Source: CAD feature listing. Evaluate the final solid. Frame: model axes, mm. A direction names the side the tool comes from. Coordinates: 2 decimals unless noted, no trailing zeros. Order: outer loops, then holes, each group sorted by start corner. A loop starts at its lowest first (then second) coordinate and runs counter-clockwise, first axis right, second up.
```python
from build123d import *

# Parameters (mm, degrees)
TOP_CHAMFER_SIZE   = 1.5
BACK_CHAMFER_SIZE  = 2
BACK_CHAMFER_SIZE2 = 11.342563639
WIRE_START         = -3.75
SKETCH8_W          = 5
SKETCH8_H          = 8.066717416
WIRE_HOLE_DEPTH    = 3.75
SKETCH9_R          = 0.875
FRONT_HOLES_DEPTH  = 6
SKETCH10_R         = 1.375
BACK_HOLES_DEPTH   = 5
SKETCH14_W         = 0.21
SKETCH14_H         = 7.302222222


with BuildPart() as part:
    # Sketch7 → Base Motor Housing (revolve)
    with BuildSketch(Plane.XY, mode=Mode.PRIVATE) as base_motor_housing_sk:
        Polygon((-38, 38.06), (-35, 38.06), (-35, 35.81), (-30.0375, 35.81), (-30.0375, 3.255), (-29.075, 3.255), (-29.075, 0), (-9, 0), (-9, -2.94), (-12, -2.94), (-12, -13.19), (-38, -13.19), (-38, 3.255), align=None)
    revolve(base_motor_housing_sk.sketch.rotate(Axis((0, -30.231871117, 0), (0, 1, 0)), 270), axis=Axis((0, -30.231871117, 0), (0, 1, 0)))

    # Top Chamfer
    top_chamfer_edges = [part.edges().sort_by_distance(p)[0] for p in [
        (0, 35.81, 30.0375),
    ]]
    chamfer(top_chamfer_edges, length=TOP_CHAMFER_SIZE)

    # Back Chamfer
    back_chamfer_edges = [part.edges().sort_by_distance(p)[0] for p in [
        (0, 0, 9),
    ]]
    back_chamfer_side = [part.faces().sort_by_distance(p)[0] for p in [
        (0, -1.47, 9),
    ]]
    chamfer(back_chamfer_edges, length=BACK_CHAMFER_SIZE, length2=BACK_CHAMFER_SIZE2, reference=back_chamfer_side[0])

    # Sketch8 → Wire Hole (cut)
    with BuildSketch(Plane(origin=(0, 38.06, 0), x_dir=(1, 0, 0), z_dir=(0, 1, 0)).offset(WIRE_START)):
        with Locations((0, -33.966641292)):
            Rectangle(SKETCH8_W, SKETCH8_H)
    extrude(amount=WIRE_HOLE_DEPTH, mode=Mode.SUBTRACT)

    # Sketch9 → Front-Holes (cut)
    with BuildSketch(Plane(origin=(0, 35.81, 0), x_dir=(1, 0, 0), z_dir=(0, 1, 0))):
        with Locations(Location((-33.26875, 0, 0), (0, 0, 270))):
            Circle(SKETCH9_R)
        with Locations(Location((-16.634375, 28.811582652, 0), (0, 0, 270))):
            Circle(SKETCH9_R)
        with Locations(Location((16.634375, 28.811582652, 0), (0, 0, 270))):
            Circle(SKETCH9_R)
        with Locations(Location((33.26875, 0, 0), (0, 0, 270))):
            Circle(SKETCH9_R)
        with Locations(Location((16.634375, -28.811582652, 0), (0, 0, 270))):
            Circle(SKETCH9_R)
        with Locations(Location((-16.634375, -28.811582652, 0), (0, 0, 270))):
            Circle(SKETCH9_R)
    extrude(amount=-FRONT_HOLES_DEPTH, mode=Mode.SUBTRACT)

    # Sketch10 → Back-Holes (cut)
    with BuildSketch(Plane.XZ.offset(13.19)):
        with Locations(Location((-25, 0, 0), (0, 0, 270))):
            Circle(SKETCH10_R)
        with Locations(Location((-12.5, 21.650635095, 0), (0, 0, 270))):
            Circle(SKETCH10_R)
        with Locations(Location((12.5, 21.650635095, 0), (0, 0, 270))):
            Circle(SKETCH10_R)
        with Locations(Location((25, 0, 0), (0, 0, 270))):
            Circle(SKETCH10_R)
        with Locations(Location((12.5, -21.650635095, 0), (0, 0, 270))):
            Circle(SKETCH10_R)
        with Locations(Location((-12.5, -21.650635095, 0), (0, 0, 270))):
            Circle(SKETCH10_R)
    extrude(amount=-BACK_HOLES_DEPTH, mode=Mode.SUBTRACT)

    # Sketch11 → Lightening Cut (revolve, cut)
    with BuildSketch(Plane.XY, mode=Mode.PRIVATE) as lightening_cut_sk:
        Polygon((29, -13.19), (29, -5.69), (35, -2.225898385), (35, 25.274101615), (38, 28.06), (38, -13.19), align=None)
    revolve(lightening_cut_sk.sketch.rotate(Axis((0, 0, 0), (0, -1, 0)), 90), axis=Axis((0, 0, 0), (0, -1, 0)), mode=Mode.SUBTRACT)

    # Sketch12 → Undercut for Stator (revolve, cut)
    with BuildSketch(Plane.XY, mode=Mode.PRIVATE) as undercut_for_stator_sk:
        Polygon((-30.0375, 3.255), (-30.7875, 3.255), (-30.0375, 3.688012702), align=None)
    revolve(undercut_for_stator_sk.sketch.rotate(Axis((0, -4.281937273, 0), (0, 1, 0)), 270), axis=Axis((0, -4.281937273, 0), (0, 1, 0)), mode=Mode.SUBTRACT)

    # Sketch14 → Adhesive Trench (revolve, cut)
    with BuildSketch(Plane.XY, mode=Mode.PRIVATE) as adhesive_trench_sk:
        with Locations((-30.1425, 24.433611111)):
            Rectangle(SKETCH14_W, SKETCH14_H)
        with Locations((-30.1425, 13.131388889)):
            Rectangle(SKETCH14_W, SKETCH14_H)
    revolve(adhesive_trench_sk.sketch.rotate(Axis((0, -10.498587948, 0), (0, 1, 0)), 270), axis=Axis((0, -10.498587948, 0), (0, 1, 0)), mode=Mode.SUBTRACT)


solid = part.part
```
1. Draft query along Z for faces 1 (the face through (13, -8.19, -22)), 2 (the face through (34.168, 11.717, -7.587)), 3 (the face through (2.5, 35, 35)). Return one class per face: released by +Z, released by -Z, zero draft, split by the parting line, or undercut.
Findings:
face 1: undercut
face 2: split by the parting line
face 3: zero draft
2. Section query A-A on y = 8.5. Return loops of the section in (x, z) (1 decimal).
Findings:
outline: circle Ø70 at (0, 0); hole circle Ø60.1 at (0, 0)
3. Access query for faces 4 (the face through (-2.5, 35, 35)), 5 (the face through (13, -8.19, 22)), 6 (the face through (-29.99, 13.18, 3.94)), 7 (the face through (-31.3, 35.81, 5.3)). Directions: +Z, -Z, +X, -X, +Y, -Y. A direction counts if a zero-diameter tool reaches every point of the face in a straight line with its end or side. Return the directions, or none.
Findings:
face 4: +Z, +Y
face 5: -Y
face 6: none
face 7: +Y
4. Pin query (flat end, axial travel): P1, Ø2, axis at x = 12.5, z = 21.65, coming from the +Y side; P2, Ø18.5, axis at x = 5.5, z = 7.5, coming from the +Y side; P3, Ø1.5, axis at x = -20.5, y = 9, coming from the -Z side. Return the tip coordinate at first contact, or that it passes through.
Findings:
P1: stops at y = 0
P2: stops at y = -0.32
P3: stops at z = -28.9
5. Ray query, line 1 (X direction, y = -9, z = 0) (3 decimals); line 2 (X direction, y = 34, z = -27.5); line 3 (Z direction, x = -2, y = 25). Return the intervals inside material, ascending.
Findings:
line 1: x = -29 to -26.375, -23.625 to -12, 12 to 23.625, 26.375 to 29
line 2: x = -26.22 to -12.08, 12.08 to 26.22
line 3: z = -34.94 to -30.18, 30.18 to 34.94
